from build123d import *

# Parameters (mm, degrees)
BOSS_EXTRUDE4_DEPTH = 5
SKETCH6_W           = 70
SKETCH6_H           = 70
BOSS_EXTRUDE5_DEPTH = 30
SKETCH8_R           = 3
CUT_EXTRUDE1_DEPTH  = 2
CUT_EXTRUDE2_START  = -30
CUT_EXTRUDE2_DEPTH  = 30
SKETCH10_W          = 140
SKETCH10_H          = 70
BOSS_EXTRUDE6_DEPTH = 2.5
FILLET1_R           = 10
SKETCH11_W          = 202.57423707
SKETCH11_H          = 181.335779968
CUT_EXTRUDE3_DEPTH  = 27.5
SKETCH12_W          = 1.775
SKETCH12_H          = 55
BOSS_EXTRUDE9_DEPTH = 27.5
CUT_EXTRUDE4_DEPTH  = 15
CHAMFER2_SIZE       = 1.25
CHAMFER4_SIZE       = 1.25
CHAMFER5_SIZE       = 1.25


with BuildPart() as part:
    # Sketch5 → Boss-Extrude4 (new body)
    with BuildSketch(Plane(origin=(0, 0, 0), x_dir=(1, 0, 0), z_dir=(0, 1, 0))):
        with BuildLine():
            Line((-22.5, -32.5), (22.5, -32.5))
            ThreePointArc((22.5, -32.5), (29.571067812, -29.571067812), (32.5, -22.5))
            Line((32.5, -22.5), (32.5, 22.5))
            ThreePointArc((32.5, 22.5), (29.571067812, 29.571067812), (22.5, 32.5))
            Line((22.5, 32.5), (-22.5, 32.5))
            ThreePointArc((-22.5, 32.5), (-29.571067812, 29.571067812), (-32.5, 22.5))
            Line((-32.5, 22.5), (-32.5, -22.5))
            ThreePointArc((-32.5, -22.5), (-29.571067812, -29.571067812), (-22.5, -32.5))
        make_face()
    extrude(amount=BOSS_EXTRUDE4_DEPTH)

    # Sketch6 → Boss-Extrude5 (add)
    with BuildSketch(Plane(origin=(0, 5, 0), x_dir=(1, 0, 0), z_dir=(0, 1, 0))):
        Rectangle(SKETCH6_W, SKETCH6_H)
    extrude(amount=BOSS_EXTRUDE5_DEPTH)

    # Sketch8 → Cut-Extrude1 (cut)
    with BuildSketch(Plane.XZ):
        with Locations(Location((26.037533906, -26.035533906, 0), (0, 0, 270))):
            Circle(SKETCH8_R)
        with Locations(Location((26.036533906, 26.036533906, 0), (0, 0, 270))):
            Circle(SKETCH8_R)
        with BuildLine():
            ThreePointArc((-23.035533906, 26.035533906), (-24.887483609, 28.807172503), (-28.156854249, 28.156854249))
            Line((-28.156854249, 28.156854249), (-23.914213562, 23.914213562))
            ThreePointArc((-23.914213562, 23.914213562), (-23.263895308, 24.887483609), (-23.035533906, 26.035533906))
        make_face()
        with BuildLine():
            Line((-23.914213562, 23.914213562), (-28.156854249, 28.156854249))
            ThreePointArc((-28.156854249, 28.156854249), (-28.156854249, 23.914213562), (-23.914213562, 23.914213562))
        make_face()
        with Locations(Location((-26.034533906, -26.036533906, 0), (0, 0, 270))):
            Circle(SKETCH8_R)
    extrude(amount=-CUT_EXTRUDE1_DEPTH, mode=Mode.SUBTRACT)

    # Mirror1: part across plane


with BuildPart() as part_1:
    add(part.part)
    add(part.part.mirror(Plane(origin=(-35, 35, -35), x_dir=(0, 0, 1), z_dir=(1, 0, 0))))

    # Sketch9 → Cut-Extrude2 (cut)
    with BuildSketch(Plane(origin=(0, 35, 0), x_dir=(1, 0, 0), z_dir=(0, 1, 0)).offset(CUT_EXTRUDE2_START)):
        with BuildLine():
            Line((22.5, 32.5), (-92.5, 32.5))
            ThreePointArc((-92.5, 32.5), (-99.571067812, 29.571067812), (-102.5, 22.5))
            Line((-102.5, 22.5), (-102.5, -22.5))
            ThreePointArc((-102.5, -22.5), (-99.571067812, -29.571067812), (-92.5, -32.5))
            Line((-92.5, -32.5), (22.5, -32.5))
            ThreePointArc((22.5, -32.5), (29.571067812, -29.571067812), (32.5, -22.5))
            Line((32.5, -22.5), (32.5, 22.5))
            ThreePointArc((32.5, 22.5), (29.571067812, 29.571067812), (22.5, 32.5))
        make_face()
    extrude(amount=CUT_EXTRUDE2_DEPTH, mode=Mode.SUBTRACT)


with BuildPart() as cut_extrude2_piece_1:
    # of the separate pieces the step leaves, piece 1, a body of its own (cut_extrude2_pieces)
    add(part_1.part.solids().sort_by_distance((35, 5, -35))[0])



with BuildPart() as cut_extrude2_piece_2:
    # of the separate pieces the step leaves, piece 2, a body of its own (cut_extrude2_pieces)
    add(part_1.part.solids().sort_by_distance((-22.5, 0, 32.5))[0])


with BuildPart() as cut_extrude2_piece_3:
    # of the separate pieces the step leaves, piece 3, a body of its own (cut_extrude2_pieces)
    add(part_1.part.solids().sort_by_distance((-92.5, 0, -32.5))[0])


with BuildPart() as cut_extrude2_piece_1_1:
    add(cut_extrude2_piece_1.part)

    add(cut_extrude2_piece_2.part)  # Boss-Extrude6 merges Cut-Extrude2 piece 2

    add(cut_extrude2_piece_3.part)  # Boss-Extrude6 merges Cut-Extrude2 piece 3
    # Sketch10 → Boss-Extrude6 (add)
    with BuildSketch(Plane.XZ.offset(-5)):
        with Locations((-35, 0)):
            Rectangle(SKETCH10_W, SKETCH10_H)
    extrude(amount=-BOSS_EXTRUDE6_DEPTH)

    # Fillet1
    fillet1_edges = [cut_extrude2_piece_1_1.edges().sort_by_distance(p)[0] for p in [
        (35, 20, 35),
        (35, 20, -35),
        (-105, 20, 35),
        (-105, 20, -35),
    ]]
    fillet(fillet1_edges, radius=FILLET1_R)

    # Sketch11 → Cut-Extrude3 (cut)
    with BuildSketch(Plane(origin=(0, 35, 0), x_dir=(1, 0, 0), z_dir=(0, 1, 0))):
        with Locations((-35, 32.5)):
            Rectangle(SKETCH11_W, SKETCH11_H)
    extrude(amount=-CUT_EXTRUDE3_DEPTH, mode=Mode.SUBTRACT)

    # Sketch12 → Boss-Extrude9 (add)
    with BuildSketch(Plane(origin=(0, 7.5, 0), x_dir=(1, 0, 0), z_dir=(0, 1, 0))):
        with BuildLine():
            Line((-105, 25), (-105, -25))
            ThreePointArc((-105, -25), (-102.071067812, -32.071067812), (-95, -35))
            Line((-95, -35), (25, -35))
            ThreePointArc((25, -35), (32.071067812, -32.071067812), (35, -25))
            Line((35, -25), (35, 25))
            ThreePointArc((35, 25), (32.071067812, 32.071067812), (25, 35))
            Line((25, 35), (-95, 35))
            ThreePointArc((-95, 35), (-102.071067812, 32.071067812), (-105, 25))
        make_face()
        with Locations((-85, 0)):
            Rectangle(SKETCH12_W, SKETCH12_H, mode=Mode.SUBTRACT)
        with Locations((-75, 0)):
            Rectangle(SKETCH12_W, SKETCH12_H, mode=Mode.SUBTRACT)
        with Locations((-65, 0)):
            Rectangle(SKETCH12_W, SKETCH12_H, mode=Mode.SUBTRACT)
        with Locations((-55, 0)):
            Rectangle(SKETCH12_W, SKETCH12_H, mode=Mode.SUBTRACT)
        with Locations((-45, 0)):
            Rectangle(SKETCH12_W, SKETCH12_H, mode=Mode.SUBTRACT)
        with Locations((-35, 0)):
            Rectangle(SKETCH12_W, SKETCH12_H, mode=Mode.SUBTRACT)
        with Locations((-95, 0)):
            Rectangle(SKETCH12_W, SKETCH12_H, mode=Mode.SUBTRACT)
        with Locations((-25, 0)):
            Rectangle(SKETCH12_W, SKETCH12_H, mode=Mode.SUBTRACT)
        with Locations((-15, 0)):
            Rectangle(SKETCH12_W, SKETCH12_H, mode=Mode.SUBTRACT)
        with Locations((-5, 0)):
            Rectangle(SKETCH12_W, SKETCH12_H, mode=Mode.SUBTRACT)
        with Locations((5, 0)):
            Rectangle(SKETCH12_W, SKETCH12_H, mode=Mode.SUBTRACT)
        with Locations((15, 0)):
            Rectangle(SKETCH12_W, SKETCH12_H, mode=Mode.SUBTRACT)
        with Locations((25, 0)):
            Rectangle(SKETCH12_W, SKETCH12_H, mode=Mode.SUBTRACT)
    extrude(amount=BOSS_EXTRUDE9_DEPTH)

    # Sketch13 → Cut-Extrude4 (cut)
    with BuildSketch(Plane(origin=(0, 35, 0), x_dir=(1, 0, 0), z_dir=(0, 1, 0))):
        with BuildLine():
            Line((32.5, -25), (32.5, 25))
            ThreePointArc((32.5, 25), (30.303300859, 30.303300859), (25, 32.5))
            Line((25, 32.5), (-95, 32.5))
            ThreePointArc((-95, 32.5), (-100.303300859, 30.303300859), (-102.5, 25))
            Line((-102.5, 25), (-102.5, -25))
            ThreePointArc((-102.5, -25), (-100.303300859, -30.303300859), (-95, -32.5))
            Line((-95, -32.5), (25, -32.5))
            ThreePointArc((25, -32.5), (30.303300859, -30.303300859), (32.5, -25))
        make_face()
    extrude(amount=-CUT_EXTRUDE4_DEPTH, mode=Mode.SUBTRACT)

    # Chamfer2
    chamfer2_edges = [cut_extrude2_piece_1_1.edges().sort_by_distance(p)[0] for p in [
        (30.303300859, 20, -30.303300859),
        (32.5, 20, 0),
        (30.303300859, 20, 30.303300859),
        (-35, 20, 32.5),
        (-100.303300859, 20, 30.303300859),
        (-102.5, 20, 0),
        (-100.303300859, 20, -30.303300859),
        (-35, 20, -32.5),
        (30.303300859, 35, -30.303300859),
        (-35, 35, -32.5),
        (-100.303300859, 35, -30.303300859),
        (-102.5, 35, 0),
        (-100.303300859, 35, 30.303300859),
        (-35, 35, 32.5),
        (30.303300859, 35, 30.303300859),
        (32.5, 35, 0),
    ]]
    chamfer(chamfer2_edges, length=CHAMFER2_SIZE)

    # Chamfer4
    chamfer4_edges = [cut_extrude2_piece_1_1.edges().sort_by_distance(p)[0] for p in [
        (-29.571067812, 0, 29.571067812),
        (0, 0, 32.5),
        (29.571067812, 0, 29.571067812),
        (32.5, 0, 0),
        (29.571067812, 0, -29.571067812),
        (0, 0, -32.5),
        (-29.571067812, 0, -29.571067812),
        (-32.5, 0, 0),
        (-40.428932188, 0, 29.571067812),
        (-70, 0, 32.5),
        (-99.571067812, 0, 29.571067812),
        (-102.5, 0, 0),
        (-99.571067812, 0, -29.571067812),
        (-70, 0, -32.5),
        (-40.428932188, 0, -29.571067812),
        (-37.5, 0, 0),
        (-35, 5, -35),
        (-35, 5, 35),
        (-105, 5, 0),
        (35, 5, 0),
        (-102.071067812, 5, -32.071067812),
        (-102.071067812, 5, 32.071067812),
        (32.071067812, 5, 32.071067812),
        (32.071067812, 5, -32.071067812),
    ]]
    chamfer(chamfer4_edges, length=CHAMFER4_SIZE)

    # Chamfer5
    chamfer5_edges = [cut_extrude2_piece_1_1.edges().sort_by_distance(p)[0] for p in [
        (25.8875, 20, 0),
        (-94.1125, 20, 0),
        (-95.8875, 20, 0),
        (-84.1125, 20, 0),
        (-85.8875, 20, 0),
        (-74.1125, 20, 0),
        (-75.8875, 20, 0),
        (-64.1125, 20, 0),
        (-65.8875, 20, 0),
        (-54.1125, 20, 0),
        (-55.8875, 20, 0),
        (-44.1125, 20, 0),
        (-45.8875, 20, 0),
        (-34.1125, 20, 0),
        (-35.8875, 20, 0),
        (-24.1125, 20, 0),
        (-25.8875, 20, 0),
        (-14.1125, 20, 0),
        (-15.8875, 20, 0),
        (-4.1125, 20, 0),
        (-5.8875, 20, 0),
        (5.8875, 20, 0),
        (4.1125, 20, 0),
        (15.8875, 20, 0),
        (14.1125, 20, 0),
        (24.1125, 20, 0),
    ]]
    chamfer(chamfer5_edges, length=CHAMFER5_SIZE)


solid = cut_extrude2_piece_1_1.part
Source: CAD feature listing. Evaluate the final solid. Frame: model axes, mm. A direction names the side the tool comes from. Coordinates: 2 decimals unless noted, no trailing zeros. Loops run counter-clockwise (first coordinate to the right, second up) from the corner with the lowest first, then second, coordinate; pieces in that order, holes last. Notation, with made-up numbers: (6.25, 21) -> (43.25, 21) arc R22 cw to (43.25, 33) -> close; hole circle Ø6 at (3.25, 25.5). An arc over 180 degrees is marked (long way). Answer in a Markdown table with one row per item. Add a question column.
Q1. Reachability of faces 1 (the face through (-29.65, 3.1, 29.49)), 2 (the face through (-26, 2, -26)), 3 (the face through (0, 3, -32.5)), 4 (the face through (-99.71, 20.34, 29.61)) from +Z, -Z, +X, -X, +Y, -Y: full face, straight path, thin tool, end or side. Return the list, or none.
Q2. Contact query for flat-ended pins moving along their axis: pin 1 Ø1.1 at (y, z) = (2, 2) entering from +X; pin 2 Ø0.9 at (x, z) = (-54.5, 9.5) entering from +Y; pin 3 Ø7 at (x, z) = (-96.04, -26.04) entering from +Y. Output: stop coordinate, or through.
Q3. Ray query, line 1 along Z through (x, y) = (-10, 27); line 2 along X through (y, z) = (25, -14); line 3 along X through (y, z) = (2.5, -3.5). Return the intervals inside material, ascending.
Q4. Pull-direction query (X, two-part tool) for faces 5 (the face through (15, 14, 27.5)), 6 (the face through (0, 3, 32.5)); classes: pulls with the +X half, pulls with the -X half, needs draft (parallel to the pull), parting line crosses it, or undercut.
Q5. Section A-A on y = 29. Return the cut outline in (x, z).
Q6. Section C-C on y = 16.5. Give the number of separate pieces and of enclosed holes in the cut face, and give its area (3 significant figures).
Q7. Section B-B on x = 9. Return the cut outline in (y, z), and give its area (3 significant figures).
Computed values:
| question | item | result |
|---|---|---|
| 1 | face 1 | +Z, -Y |
| 1 | face 2 | -Y |
| 1 | face 3 | -Z, +X, -X, -Y |
| 1 | face 4 | +Y |
| 2 | pin 1 | stops at x = 32.5 |
| 2 | pin 2 | stops at y = 18.81 |
| 2 | pin 3 | stops at y = 20 |
| 3 | line 1 | z = -35 to -32.5, 32.5 to 35 |
| 3 | line 2 | x = -105 to -102.5, 32.5 to 35 |
| 3 | line 3 | x = -102.5 to -37.5, -32.5 to 32.5 |
| 4 | face 5 | undercut |
| 4 | face 6 | needs draft |
| 5 | outline | (-105, -25) arc R10 ccw to (-95, -35) -> (25, -35) arc R10 ccw to (35, -25) -> (35, 25) arc R10 ccw to (25, 35) -> (-95, 35) arc R10 ccw to (-105, 25) -> close; hole (-102.5, -25) arc R7.5 ccw to (-95, -32.5) -> (25, -32.5) arc R7.5 ccw to (32.5, -25) -> (32.5, 25) arc R7.5 ccw to (25, 32.5) -> (-95, 32.5) arc R7.5 ccw to (-102.5, 25) -> close |
| 6 | separate pieces | 1 |
| 6 | enclosed holes | 13 |
| 6 | area | 8,450 mm^2 |
| 7 | outline | (0, -31.25) -> (1.25, -32.5) -> (5, -32.5) -> (5, -33.75) -> (6.25, -35) -> (35, -35) -> (35, -33.75) -> (33.75, -32.5) -> (21.25, -32.5) -> (20, -31.25) -> (20, 31.25) -> (21.25, 32.5) -> (33.75, 32.5) -> (35, 33.75) -> (35, 35) -> (6.25, 35) -> (5, 33.75) -> (5, 32.5) -> (1.25, 32.5) -> (0, 31.25) -> close |
| 7 | area | 1,450 mm^2 |
